Read the model definition and answer for the solid it produces. Units are mm, in the model's axes. A direction names the side the tool comes from. Give positions to 0.01 mm unless a question says otherwise; leave off trailing zeros. Write each loop counter-clockwise with the first axis right and the second up, starting at its lowest first coordinate (ties: lowest second). Pieces come first, ordered by that corner, then holes. Notation, with made-up numbers: M -29,80 L 1,80 A19 cw 1,117 Z; hole C 63,43 d8. An arc over 180 degrees is marked long. Put each result on its own line as item: value.
from build123d import *

# Parameters (mm, degrees)
SKETCH1_R           = 2
SKETCH1_R_2         = 4
SKETCH1_R_3         = 11
BOSS_EXTRUDE1_DEPTH = 6


with BuildPart() as part:
    # Sketch1 → Boss-Extrude1 (new body)
    with BuildSketch(Plane.XY):
        Polygon((-194, 30), (-194, -30), (194, -30), (194, 30), (164, 30), (164, 23), (144, 23), (144, 30), align=None)
        with Locations((-185, -10)):
            Circle(SKETCH1_R, mode=Mode.SUBTRACT)
        with Locations((185, -10)):
            Circle(SKETCH1_R, mode=Mode.SUBTRACT)
        with Locations((-185, 10)):
            Circle(SKETCH1_R, mode=Mode.SUBTRACT)
        with Locations((-60, 15)):
            Circle(SKETCH1_R_2, mode=Mode.SUBTRACT)
        Circle(SKETCH1_R_3, mode=Mode.SUBTRACT)
        with Locations((185, 10)):
            Circle(SKETCH1_R, mode=Mode.SUBTRACT)
        with Locations((60, 15)):
            Circle(SKETCH1_R_2, mode=Mode.SUBTRACT)
    extrude(amount=BOSS_EXTRUDE1_DEPTH)


solid = part.part
(1) Which of the six approach directions +Z, -Z, +X, -X, +Y, -Y give full straight-line access (tool end or side, diameter ignored) to faces 1 (the face through (179, 30, 3)), 2 (the face through (164, 27, 3))?
Result:
face 1: +Z, -Z, +X, -X, +Y
face 2: +Z, -Z, +Y
(2) Straight lines are drawn through the part: line 1 along Y through (x, z) = (-185, 1.5); line 2 along X through (y, z) = (-9, 1.35); line 3 along X through (y, z) = (16.5, 4.85). For each, find the intervals that lie inside material, in ascending order. Write a range as from..to.
Result:
line 1: y = -30..-12, -8..8, 12..30
line 2: x = -194..-186.73, -183.27..-6.32, 6.32..183.27, 186.73..194
line 3: x = -194..-63.71, -56.29..56.29, 63.71..194
(3) Section A-A on x = 0 is taken. Determine the outline of the cut face in (y, z), and give its area (3 significant figures).
Result:
outline: M -30,0 L -11,0 L -11,6 L -30,6 Z; M 11,0 L 30,0 L 30,6 L 11,6 Z
area: 228 mm²
(4) Section B-B on z = 3.9 is taken. Determine the outline of the cut face in (x, y), and give its area (3 significant figures).
Result:
outline: M -194,-30 L 194,-30 L 194,30 L 164,30 L 164,23 L 144,23 L 144,30 L -194,30 Z; hole C -185,-10 d4; hole C -185,10 d4; hole C -60,15 d8; hole C 0,0 d22; hole C 60,15 d8; hole C 185,-10 d4; hole C 185,10 d4
area: 22,600 mm²
(5) Given pin 1 Ø10 at (x, y) = (-149.5, -16) entering from -Z, flat-ended and moving along its own axis, determine where the tip first touches the part or whether it passes through.
Result:
pin 1: stops at z = 0
(6) Section C-C on y = 0 is taken. Determine the outline of the cut face in (x, z), and give its area (3 significant figures).
Result:
outline: M -194,0 L -11,0 L -11,6 L -194,6 Z; M 11,0 L 194,0 L 194,6 L 11,6 Z
area: 2,200 mm²
